Build history of the part. All positions in model axes, mm. Coordinates: 2 decimals unless noted, no trailing zeros. Order: outer loops, then holes, each group sorted by start corner. A loop starts at its lowest first (then second) coordinate and runs counter-clockwise, first axis right, second up. Notation, with made-up numbers: (-27.5, -30.75) - (26.5, -30.75) arc R23 cw to (26.5, -13.75) - close; hole circle Ø10 at (-9, 36). An arc over 180 degrees is marked (long way). One line per item, written item: value.
from build123d import *

# Parameters (mm, degrees)
BOSS_EXTRUDE1_DEPTH      = 2
M2_CLEARANCE_HOLE1_D     = 2
M2_CLEARANCE_HOLE1_DEPTH = 2
M2_CLEARANCE_HOLE1_TIP   = 0.600860619


with BuildPart() as part:
    # Sketch1 → Boss-Extrude1 (new body)
    with BuildSketch(Plane(origin=(0, 0, 0), x_dir=(1, 0, 0), z_dir=(0, 1, 0))):
        Polygon((98, 45), (136, 45), (136, 0), (98, 0), (98, -17.5), (38, -17.5), (38, 0), (0, 0), (0, 45), (38, 45), (38, 62.5), (98, 62.5), align=None)
    extrude(amount=BOSS_EXTRUDE1_DEPTH)

    # M2 Clearance Hole1
    with Locations(Plane(origin=(0, 2, 0), x_dir=(1, 0, 0), z_dir=(0, 1, 0))):
        with Locations((2.5, 5), (2.5, 40), (133.5, 40), (133.5, 5)):
            Hole(M2_CLEARANCE_HOLE1_D / 2, depth=M2_CLEARANCE_HOLE1_DEPTH)
            with Locations((0, 0, -(M2_CLEARANCE_HOLE1_DEPTH + M2_CLEARANCE_HOLE1_TIP / 2))):  # 118° drill point
                Cone(0, M2_CLEARANCE_HOLE1_D / 2, M2_CLEARANCE_HOLE1_TIP, mode=Mode.SUBTRACT)


solid = part.part
1. Band-saw the part on C-C, the plane x = 12. Give the cut face in (y, z), and give its area (3 significant figures).
Values found:
outline: (0, -45) - (2, -45) - (2, 0) - (0, 0) - close
area: 90.0 mm2
2. Band-saw the part on A-A, the plane y = 1.15. Give the cut face in (x, z), and give its area (3 significant figures).
Values found:
outline: (0, -45) - (38, -45) - (38, -62.5) - (98, -62.5) - (98, -45) - (136, -45) - (136, 0) - (98, 0) - (98, 17.5) - (38, 17.5) - (38, 0) - (0, 0) - close; hole circle Ø2 at (2.5, -40); hole circle Ø2 at (2.5, -5); hole circle Ø2 at (133.5, -40); hole circle Ø2 at (133.5, -5)
area: 8,210 mm2
3. Band-saw the part on B-B, the plane z = 2. Give the cut face in (x, y), and give its area (3 significant figures).
Values found:
outline: (38, 0) - (98, 0) - (98, 2) - (38, 2) - close
area: 120 mm2
4. Probe line 1 along Z through (x, y) = (133.5, 1.55); line 2 along X through (y, z) = (1.5, -5); line 3 along X through (y, z) = (1.55, -58). List the from-to ranges inside material, lowest first.
Values found:
line 1: z = -45 to -41, -39 to -6, -4 to 0
line 2: x = 0 to 1.5, 3.5 to 132.5, 134.5 to 136
line 3: x = 38 to 98
5. Flat gauge pins, fed straight in: P1, Ø0.6, axis at x = 17, y = 1, coming from the -Z side; P2, Ø1, axis at x = 109.5, y = 1.5, coming from the +Z side; P3, Ø0.6, axis at y = 1, z = -56.5, coming from the +X side. Where does each tip first touch, or does it go through?
Values found:
P1: stops at z = -45
P2: stops at z = 0
P3: stops at x = 98
